Autodesk Inventor part; units mm, degrees
ref_plane "YZ Plane" through (0, 0, 0) normal (1, 0, 0) x (0, 1, 0)
ref_plane "XZ Plane" through (0, 0, 0) normal (0, 1, 0) x (-1, 0, 0)
ref_plane "XY Plane" through (0, 0, 0) normal (0, 0, 1) x (1, 0, 0)
sketch "main" plane through (0, 0, 0) normal (0, 0, 1) x (1, 0, 0)
  circle A0 centre (38.7007, 32.2161) radius 2.3114
  circle A1 centre (29.7205, 23.2358) radius 2.3114
  circle A2 centre (13.1029, 17.5349) radius 2.1844
  circle A3 centre (22.281, -19.1287) radius 2.1844
  circle A4 centre (22.281, -19.1287) radius 6.35
  spline S0 degree 3 poles (34.2106, 36.7062) (34.5464, 37.0421) (35.2145, 37.7033) (36.4253, 38.4715) (37.8969, 38.8878) (39.5045, 38.8877) (40.9769, 38.4718) (42.187, 37.7033) (42.855, 37.0421) (43.1908, 36.7062) knots 0 0 0 0 0.123366 0.246731 0.370097 0.493463 0.616828 0.740194 0.86356 0.86356 0.86356 0.86356
  spline S1 degree 3 poles (43.1908, 36.7062) (43.5267, 36.3703) (44.188, 35.7023) (44.9562, 34.4914) (45.3725, 33.0199) (45.3723, 31.4123) (44.9564, 29.9399) (44.1879, 28.7298) (43.5267, 28.0618) (43.1908, 27.7259) knots 0 0 0 0 0.123366 0.246731 0.370097 0.493463 0.616828 0.740194 0.86356 0.86356 0.86356 0.86356
  line L0 (28.3198, -21.092) -> (45.0845, 30.4731)
  line L1 (16.2421, -17.1653) -> (28.0767, 19.2357)
  line L2 (24.0195, 11.1849) -> (0.4029, 11.1849)
  spline S2 degree 3 poles (28.5097, 13.0448) (28.2578, 12.7929) (27.7518, 12.2921) (26.7458, 11.6097) (25.4482, 11.197) (24.4945, 11.1849) (24.0195, 11.1849) knots 0 0 0 0 0.214286 0.428571 0.714286 1 1 1 1
  point P0 (28.3293, 11.5879)
  dimension "d0" = 12.7
sketch "Sketch1" plane through (0, 0, 0) normal (0, 1, 0) x (-1, 0, 0)
  circle A0 centre (22.1371, 19.4505) radius 2.3114
  circle A1 centre (-4.1584, 4.4483) radius 2.1844
  circle A2 centre (5.0197, -32.2153) radius 2.1844
  arc A3 (-1.2776, -31.3986) -> (11.0475, -34.2123) centre (5.0197, -32.2153) ccw
  line L0 (11.0475, -34.2123) -> (28.1648, 17.4535)
  line L1 (-1.2776, -31.3986) -> (2.3621, -3.335)
  line L2 (1.1026, -1.9017) -> (-29.5584, -1.9017)
  line L3 (6.1217, 12.3553) -> (17.1581, 23.3917)
  spline S0 degree 3 poles (1.4978, 10.7883) (1.9739, 10.7568) (2.9306, 10.7058) (4.2586, 11.0336) (5.3122, 11.651) (5.8525, 12.1194) (6.1217, 12.3553) knots 0 0 0 0 0.285714 0.571429 0.785714 1 1 1 1
  line L4 (-16.8584, 10.7983) -> (1.4978, 10.7883)
  arc A4 (2.3621, -3.335) -> (1.1026, -1.9017) centre (1.1026, -3.1717) ccw
  line L5 (-16.8584, 10.7983) -> (-29.5584, 10.7983)
  circle A5 centre (-29.5584, 4.4483) radius 2.1844
  arc A6 (28.1648, 17.4535) -> (17.1581, 23.3917) centre (22.1371, 19.4505) ccw
  arc A7 (-29.5584, 10.7983) -> (-29.5584, -1.9017) centre (-29.5584, 4.4483) ccw
  circle A8 centre (13.1568, 10.4703) radius 2.0955
  line L6 (-29.5584, 4.4483) -> (7.1348, 4.4483)
  line L7 (7.1348, 4.4483) -> (22.1371, 19.4505)
  dimension "d2" = 12.7
  dimension "d3" = 1.27
  dimension "d10" = 6.35
  dimension "d15" = 135
extrude "Extrusion1" add sketch "Sketch1" along normal blind 1.5875
equation "\"BendRadius\" = Thickness"
equation "\"BendReliefWidth\" = Thickness"
equation "\"BendReliefDepth\" = 0.5 * Thickness"
equation "\"CornerReliefSize\" = 4 * Thickness"
equation "\"MinimumRemnant\" = 2 * Thickness"
equation "\"TransitionRadius\" = BendRadius"
equation "\"JacobiRadiusSize\" = BendRadius"
equation "\"GapSize\" = Thickness"
properties part number "join-gusset_offset" material "Acetal Resin, Black"
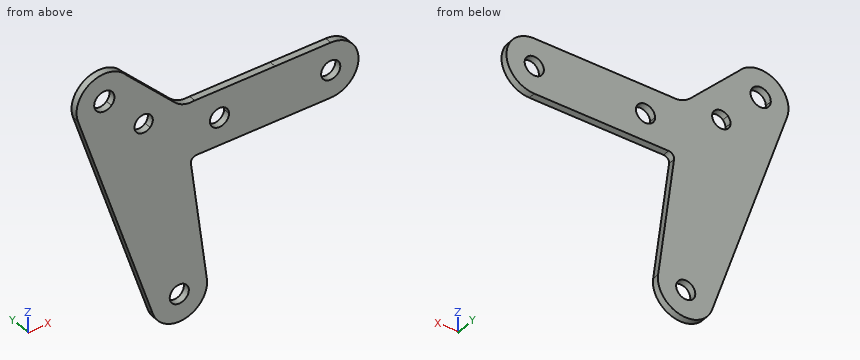
Check sheet for the modelled part. Datum: model origin and axes. Units: mm. Coordinates: 2 decimals unless noted, no trailing zeros. Write each loop counter-clockwise with the first axis right and the second up, starting at its lowest first coordinate (ties: lowest second). Pieces come first, ordered by that corner, then holes. Notation, with made-up numbers: (44.25, 22) - (50.25, 22) arc R35 cw to (50.25, 57) - close; hole circle Ø5 at (13, 79). An arc over 180 degrees is marked (long way). One line per question, with ' | ' between items.
Item 1: Sectioned sample at D-D on y = 0.35. Give the number of separate pieces and of enclosed holes in the cut face, plus the area to 3 significant figures.
Determined:
separate pieces: 1 | enclosed holes: 5 | area: 1,450 mm2
Item 2: Sectioned sample at B-B on x = 0.5. Record the boundary of the cut face in (y, z), plus the area to 3 significant figures.
Determined:
outline: (0, -35.35) - (1.59, -35.35) - (1.59, -25.4) - (0, -25.4) - close; (0, -1.9) - (1.59, -1.9) - (1.59, 10.79) - (0, 10.79) - close | area: 35.9 mm2
Item 3: Sectioned sample at C-C on x = 21.5. Record the boundary of the cut face in (y, z).
Determined:
outline: (0, -1.9) - (1.59, -1.9) - (1.59, 10.8) - (0, 10.8) - close
Item 4: Gauge pin test, flat ends, axial feed: P1, Ø4, axis at x = 29.56, z = 4.45, coming from the -Y side; P2, Ø0.5, axis at x = 21.5, y = 1, coming from the +Z side. Record the tip position at first contact, or that the pin passes through.
Determined:
P1: passes through | P2: stops at z = 10.8
Item 5: Sectioned sample at A-A on z = 5.5. Record the boundary of the cut face in (x, y), plus the area to 3 significant figures.
Determined:
outline: (-24.2, 0) - (2.24, 0) - (2.24, 1.59) - (-24.2, 1.59) - close; (6.07, 0) - (27.64, 0) - (27.64, 1.59) - (6.07, 1.59) - close; (31.47, 0) - (35.82, 0) - (35.82, 1.59) - (31.47, 1.59) - close | area: 83.1 mm2
Item 6: Thickness scan on line 1 (Z direction, x = 4, y = 0.65); line 2 (Z direction, x = 16.5, y = 1.2); line 3 (X direction, y = 1.3, z = 5). Record the ranges inside material, lowest first. Write a range as [from, to].
Determined:
line 1: z = [-1.9, 2.27], [6.63, 10.79] | line 2: z = [-1.9, 10.8] | line 3: x = [-24.04, 2.04], [6.27, 27.44], [31.67, 35.88]
